Model file for the job. Use its own axes, mm. Face numbers are marked on the shaded views. A direction names the side the tool comes from. Give positions to 0.01 mm unless a question says otherwise; leave off trailing zeros. Loops run counter-clockwise (first coordinate to the right, second up) from the corner with the lowest first, then second, coordinate; pieces in that order, holes last. Notation, with made-up numbers: (33.5, -7) - (56.5, -7) arc R24 ccw to (56.5, 3) - close; hole circle Ø1 at (28, -14). An arc over 180 degrees is marked (long way). Answer as CSV lines item,"result". Start each with the question number.
Item 1: Drill centre lines: L1, parallel to Z at x = -82, y = 49; L2, parallel to Y at x = -101, z = -15; L3, parallel to Y at x = -72, z = 16.5. Where is each one in solid material? Low to high. Write a range as from..to.
Item 2: Pin check, flat tips, straight feed: pin 1 (22 mm diameter, centred on x = -87.5, y = 38, fed in from -Z); pin 2 (3 mm diameter, centred on x = -59.5, y = 62.5, fed in from -Z); pin 3 (10 mm diameter, centred on x = -60.5, z = 2.5, fed in from -Y). Stop position of each tip, or through.
Item 3: Tool access for the marked faces 1, 2 and 3: list every direction of +Z, -Z, +X, -X, +Y, -Y with a clear straight run to the whole face (end or side of a thin tool).
Item 4: Saw through at D-D on z = 12.5. Give the cut face in (x, y), plus the area to 3 significant figures.
Item 5: Saw through at B-B on z = 3.5. Give the cut face in (x, y).
Item 6: Saw through at A-A on z = -11.5. Give the cut face in (x, y).
Item 7: Saw through at C-C on z = 20. Give the cut face in (x, y).
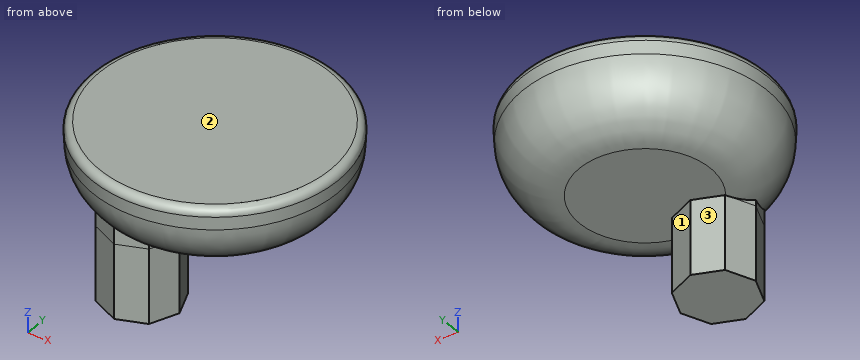
from build123d import *

# Parameters (mm, degrees)
F0_R     = 40.5620134448
F1_DEPTH = 25.4
F1_TAPER = -3
F2_R     = 2.54
F4_DEPTH = 25.4


# Not quite as in the source:
# - a fillet or chamfer that OpenCascade refuses, or shapes differently, is made with other operations: its cross-section is extruded or revolved along the edge and cut away or added


with BuildPart() as f1:
    # F0 (on Top) → F1 (new body)
    with BuildSketch(Plane.XY):
        with Locations((-84.2179358006, 32.7308289707)):
            Circle(F0_R)
    extrude(amount=F1_DEPTH, taper=F1_TAPER)

    # F2
    f2_edges = [f1.edges().sort_by_distance(p)[0] for p in [
        (-126.111107, 32.730829, 25.4),
    ]]
    fillet(f2_edges, radius=F2_R)

    # F3 (on face) → F4 (join)
    with BuildSketch(Plane(origin=(0, 0, 0), x_dir=(1, 0, 0), z_dir=(0, 0, -1))):
        Polygon((-84.1343444512, -19.9111274666), (-80.4951596333, -10.7477918976), (-84.4013240897, -1.6950429158), (-93.5646596587, 1.9441419021), (-102.6174086406, -1.9620225542), (-106.2565934585, -11.1253581232), (-102.3504290021, -20.1781071051), (-93.1870934331, -23.817291923), align=None)
    extrude(amount=F4_DEPTH)

    # F5: fillet of radius 19.304 on 1 edges, made by hand


with BuildPart() as f5_tool1:
    # F5_s2 → F5_t3 (revolve)
    with BuildSketch(Plane.XZ.offset(-32.7308289707)):
        with BuildLine():
            ThreePointArc((-42.6971898128, 18.2937067007), (-48.6867376225, 5.301373142), (-61.9747343517, 0))
            Line((-61.9747343517, 0), (-43.6559223558, 0))
            Line((-43.6559223558, 0), (-42.6971898128, 18.2937067007))
        make_face()
    revolve(axis=Axis((-84.2179358006, 32.7308289707, 0), (0, 0, 1)))

    split(bisect_by=Plane(origin=(-65.841803323, -26.1488285825, 0), x_dir=(0, 0, 1), z_dir=(0.929388426, 0.3691031748, 0)), keep=Keep.TOP)


with BuildPart() as f5_tool5:
    # F5_s6 → F5_t7 (revolve)
    with BuildSketch(Plane.XZ.offset(-32.7308289707)):
        with BuildLine():
            ThreePointArc((-42.6971898128, 18.2937067007), (-48.6867376225, 5.301373142), (-61.9747343517, 0))
            Line((-61.9747343517, 0), (-43.6559223558, 0))
            Line((-43.6559223558, 0), (-42.6971898128, 18.2937067007))
        make_face()
    revolve(axis=Axis((-84.2179358006, 32.7308289707, 0), (0, 0, 1)))

    split(bisect_by=Plane(origin=(-71.7703043479, 30.9681194552, 0), x_dir=(0, 0, 1), z_dir=(0.9181722162, -0.3961815006, 0)), keep=Keep.TOP)


with BuildPart() as f5_tool9:
    # F5_s10 → F5_t11 (revolve)
    with BuildSketch(Plane.XZ.offset(-32.7308289707)):
        with BuildLine():
            ThreePointArc((-42.6971898128, 18.2937067007), (-48.6867376225, 5.301373142), (-61.9747343517, 0))
            Line((-61.9747343517, 0), (-43.6559223558, 0))
            Line((-43.6559223558, 0), (-42.6971898128, 18.2937067007))
        make_face()
    revolve(axis=Axis((-84.2179358006, 32.7308289707, 0), (0, 0, 1)))

    split(bisect_by=Plane(origin=(-93.6255737167, 40.3984346626, 0), x_dir=(0, 0, 1), z_dir=(-0.9181722162, 0.3961815006, 0)), keep=Keep.TOP)


with BuildPart() as f5_tool13:
    # F5_s14 → F5_t15 (revolve)
    with BuildSketch(Plane.XZ.offset(-32.7308289707)):
        with BuildLine():
            ThreePointArc((-42.6971898128, 18.2937067007), (-48.6867376225, 5.301373142), (-61.9747343517, 0))
            Line((-61.9747343517, 0), (-43.6559223558, 0))
            Line((-43.6559223558, 0), (-42.6971898128, 18.2937067007))
        make_face()
    revolve(axis=Axis((-84.2179358006, 32.7308289707, 0), (0, 0, 1)))

    split(bisect_by=Plane(origin=(-12.0800640476, 30.4171637609, 0), x_dir=(0, 0, 1), z_dir=(0.3691031748, -0.929388426, 0)), keep=Keep.TOP)


with BuildPart() as f5_tool17:
    # F5_s18 → F5_t19 (revolve)
    with BuildSketch(Plane.XZ.offset(-32.7308289707)):
        with BuildLine():
            ThreePointArc((-42.6971898128, 18.2937067007), (-48.6867376225, 5.301373142), (-61.9747343517, 0))
            Line((-61.9747343517, 0), (-43.6559223558, 0))
            Line((-43.6559223558, 0), (-42.6971898128, 18.2937067007))
        make_face()
    revolve(axis=Axis((-84.2179358006, 32.7308289707, 0), (0, 0, 1)))

    split(bisect_by=Plane(origin=(-15.3930951173, -35.6743367329, 0), x_dir=(0, 0, 1), z_dir=(-0.3961815006, -0.9181722162, 0)), keep=Keep.TOP)


with BuildPart() as f5_tool21:
    # F5_s22 → F5_t23 (revolve)
    with BuildSketch(Plane.XZ.offset(-32.7308289707)):
        with BuildLine():
            ThreePointArc((-42.6971898128, 18.2937067007), (-48.6867376225, 5.301373142), (-61.9747343517, 0))
            Line((-61.9747343517, 0), (-43.6559223558, 0))
            Line((-43.6559223558, 0), (-42.6971898128, 18.2937067007))
        make_face()
    revolve(axis=Axis((-84.2179358006, 32.7308289707, 0), (0, 0, 1)))

    split(bisect_by=Plane(origin=(-87.9640523303, -34.9345979258, 0), x_dir=(0, 0, 1), z_dir=(-0.929388426, -0.3691031748, 0)), keep=Keep.TOP)


with BuildPart() as f1_1:
    add(f1.part)

    # F5_t25: cut F5_tool1, F5_tool5, F5_tool9, F5_tool13, F5_tool17, F5_tool21
    add([f5_tool1.part, f5_tool5.part, f5_tool9.part, f5_tool13.part, f5_tool17.part, f5_tool21.part], mode=Mode.SUBTRACT)


solid = f1_1.part
Responses:
1,L1,"0..25.4"
1,L2,"1.26..20.71"
1,L3,"-6.77..72.23"
2,pin 1,"z = 0"
2,pin 2,"z = 7.09"
2,pin 3,"y = 2.44"
3,face 1,"-Z, +X, +Y"
3,face 2,"+Z, +X, -X, +Y, -Y"
3,face 3,"-Z, -X, +Y"
4,outline,"circle Ø80.62 at (-84.22, 32.73)"
4,area,"5,100 mm2"
5,outline,"(-104.26, 6.1) - (-102.62, 1.96) - (-93.56, -1.94) - (-89.22, -0.22) arc R33.33 ccw (long way) to start"
6,outline,"(-106.26, 11.13) - (-102.62, 1.96) - (-93.56, -1.94) - (-84.4, 1.7) - (-80.5, 10.75) - (-84.13, 19.91) - (-93.19, 23.82) - (-102.35, 20.18) - close"
7,outline,"circle Ø83.22 at (-84.22, 32.73)"
